```python
from build123d import *

# Parameters (mm, degrees)
ESQUISSE1_R             = 37
ESQUISSE1_R_2           = 1.5
ESQUISSE1_W             = 25
ESQUISSE1_H             = 3
BOSS_EXTRU_1_DEPTH      = 2
BOSS_EXTRU_2_DEPTH      = 15
ESQUISSE3_W             = 2
ESQUISSE3_H             = 28.4
BOSS_EXTRU_3_DEPTH      = 2.25
ESQUISSE5_W             = 2
ESQUISSE5_H             = 24.4
BOSS_EXTRU_4_DEPTH      = 2.25
ESQUISSE7_W             = 33.1
ESQUISSE7_H             = 28.4
BOSS_EXTRU_5_DEPTH      = 1
ESQUISSE8_W             = 15
ESQUISSE8_H             = 15
ENL_V_MAT_EXTRU_1_DEPTH = 3
ESQUISSE9_W             = 21
ESQUISSE9_H             = 2.5
ENL_V_MAT_EXTRU_2_DEPTH = 3
ESQUISSE10_R            = 1
ENL_V_MAT_EXTRU_3_DEPTH = 19
ESQUISSE11_W            = 33.1
ESQUISSE11_H            = 28.4
ENL_V_MAT_EXTRU_4_DEPTH = 15


with BuildPart() as part:
    # Esquisse1 → Boss.-Extru.1 (new body)
    with BuildSketch(Plane.XY):
        Circle(ESQUISSE1_R)
        with Locations((0, 30)):
            Circle(ESQUISSE1_R_2, mode=Mode.SUBTRACT)
        with Locations((-22.874807889, 14.34375)):
            Circle(ESQUISSE1_R_2, mode=Mode.SUBTRACT)
        with Locations((-25.416453209, -15.9375)):
            Circle(ESQUISSE1_R_2, mode=Mode.SUBTRACT)
        with Locations((0, -27)):
            Circle(ESQUISSE1_R_2, mode=Mode.SUBTRACT)
        with Locations((25.416453209, -15.9375)):
            Circle(ESQUISSE1_R_2, mode=Mode.SUBTRACT)
        with Locations((22.874807889, 14.34375)):
            Circle(ESQUISSE1_R_2, mode=Mode.SUBTRACT)
        with Locations((0, -15.5)):
            Rectangle(ESQUISSE1_W, ESQUISSE1_H, mode=Mode.SUBTRACT)
    extrude(amount=BOSS_EXTRU_1_DEPTH)

    # Esquisse2 → Boss.-Extru.2 (add)
    with BuildSketch(Plane(origin=(0, 0, 0), x_dir=(-1, 0, 0), z_dir=(0, 0, -1))):
        Polygon((-16.75, 14.9), (-12.75, 14.9), (-12.75, -9.5), (12.35, -9.5), (12.35, 14.9), (16.35, 14.9), (16.35, -13.5), (-16.75, -13.5), align=None)
    extrude(amount=BOSS_EXTRU_2_DEPTH)

    # Esquisse3 → Boss.-Extru.3 (add)
    with BuildSketch(Plane(origin=(-12.35, 0, 0), x_dir=(0, 0, -1), z_dir=(1, 0, 0))):
        with Locations((9.625, 0.7)):
            Rectangle(ESQUISSE3_W, ESQUISSE3_H)
        with Locations((6.625, 0.7)):
            Rectangle(ESQUISSE3_W, ESQUISSE3_H)
    extrude(amount=BOSS_EXTRU_3_DEPTH)

    # Esquisse5 → Boss.-Extru.4 (add)
    with BuildSketch(Plane.ZY.offset(-12.75)):
        with Locations((-9.625, 2.7)):
            Rectangle(ESQUISSE5_W, ESQUISSE5_H)
        with Locations((-6.625, 2.7)):
            Rectangle(ESQUISSE5_W, ESQUISSE5_H)
    extrude(amount=BOSS_EXTRU_4_DEPTH)

    # Esquisse7 → Boss.-Extru.5 (add)
    with BuildSketch(Plane(origin=(0, 0, -15), x_dir=(-1, 0, 0), z_dir=(0, 0, -1))):
        with Locations((-0.2, 0.7)):
            Rectangle(ESQUISSE7_W, ESQUISSE7_H)
    extrude(amount=-BOSS_EXTRU_5_DEPTH)

    # Esquisse8 → Enlèv. mat.-Extru.1 (cut)
    with BuildSketch(Plane(origin=(0, 0, -15), x_dir=(-1, 0, 0), z_dir=(0, 0, -1))):
        Rectangle(ESQUISSE8_W, ESQUISSE8_H)
    extrude(amount=-ENL_V_MAT_EXTRU_1_DEPTH, mode=Mode.SUBTRACT)

    # Esquisse9 → Enlèv. mat.-Extru.2 (cut)
    with BuildSketch(Plane.XZ.offset(13.5)):
        with Locations((0, -5.65)):
            Rectangle(ESQUISSE9_W, ESQUISSE9_H)
    extrude(amount=-ENL_V_MAT_EXTRU_2_DEPTH, mode=Mode.SUBTRACT)

    # Esquisse10 → Enlèv. mat.-Extru.3 (cut)
    with BuildSketch(Plane.XY.offset(2)):
        with Locations((-14.35, 8.9)):
            Circle(ESQUISSE10_R)
        with Locations((-14.35, -11.5)):
            Circle(ESQUISSE10_R)
        with Locations((14.75, -11.5)):
            Circle(ESQUISSE10_R)
        with Locations((14.75, 8.9)):
            Circle(ESQUISSE10_R)
    extrude(amount=-ENL_V_MAT_EXTRU_3_DEPTH, mode=Mode.SUBTRACT)

    # Esquisse11 → Enlèv. mat.-Extru.4 (cut)
    with BuildSketch(Plane(origin=(0, 0, -15), x_dir=(-1, 0, 0), z_dir=(0, 0, -1))):
        with Locations((-0.2, 0.7)):
            Rectangle(ESQUISSE11_W, ESQUISSE11_H)
    extrude(amount=-ENL_V_MAT_EXTRU_4_DEPTH, mode=Mode.SUBTRACT)


solid = part.part
```
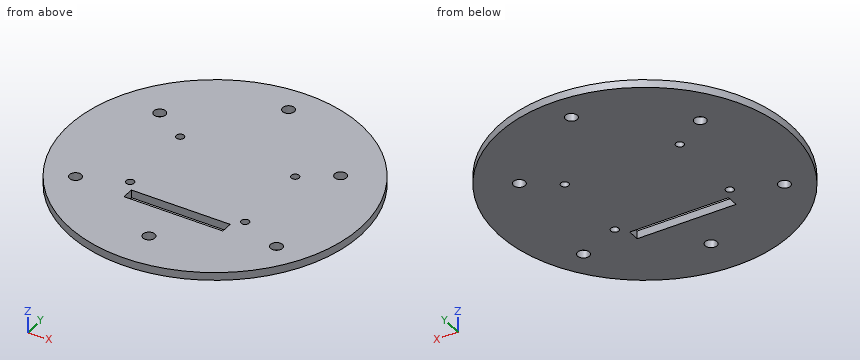
Can you work these out from the model? Positions are in its coordinate system, mm. Coordinates: 2 decimals unless noted, no trailing zeros. Write each loop counter-clockwise with the first axis right and the second up, starting at its lowest first coordinate (ties: lowest second). Pieces come first, ordered by that corner, then holes. Notation, with made-up numbers: M -22.5,29.5 L -6.5,29.5 A15 cw -6.5,49.5 Z; hole C 85.5,-34 d7. An arc over 180 degrees is marked long. Answer as CSV lines item,"result".
Item 1: Imagine slicing it at D-D on y = 30. List the corners of the cut face in (x, z) for me, plus the area to 3 significant figures.
Geometry results:
outline,"M -21.66,0 L -1.5,0 L -1.5,2 L -21.66,2 Z; M 1.5,0 L 21.66,0 L 21.66,2 L 1.5,2 Z"
area,"80.6 mm2"
Item 2: Imagine slicing it at B-B on y = 8.9. List the corners of the cut face in (x, z) for me, plus the area to 3 significant figures.
Geometry results:
outline,"M -35.91,0 L -15.35,0 L -15.35,2 L -35.91,2 Z; M -13.35,0 L 13.75,0 L 13.75,2 L -13.35,2 Z; M 15.75,0 L 35.91,0 L 35.91,2 L 15.75,2 Z"
area,"136 mm2"
Item 3: Imagine slicing it at C-C on x = -14.35. List the corners of the cut face in (y, z) for me.
Geometry results:
outline,"M -34.1,0 L -12.5,0 L -12.5,2 L -34.1,2 Z; M -10.5,0 L 7.9,0 L 7.9,2 L -10.5,2 Z; M 9.9,0 L 34.1,0 L 34.1,2 L 9.9,2 Z"
Item 4: I'm going to push flat-ended pins straight in: P1, Ø0.6, axis at x = 3, z = 1, coming from the -Y side; P2, Ø2.5, axis at x = 0, y = 30, coming from the +Z side; P3, Ø1, axis at y = -9.5, z = 2, coming from the +X side; P4, Ø0.6, axis at y = -16, z = 1, coming from the +X side. Where does each tip first touch, or does it pass through?
Geometry results:
P1,"stops at y = -36.9"
P2,"passes through"
P3,"stops at x = 35.89"
P4,"stops at x = 33.5"
Item 5: Please list where these lines run through material, in increasing order: line 1 along Y through (x, z) = (0, 1.05); line 2 along X through (y, z) = (13, 1.8); line 3 along Y through (x, z) = (-0.5, 1.3).
Geometry results:
line 1,"y = -37 to -28.5, -25.5 to -17, -14 to 28.5, 31.5 to 37"
line 2,"x = -34.64 to -23.54, -22.21 to 22.21, 23.54 to 34.64"
line 3,"y = -37 to -28.41, -25.59 to -17, -14 to 28.59, 31.41 to 37"
Item 6: Imagine slicing it at A-A on x = 0. List the corners of the cut face in (y, z) for me.
Geometry results:
outline,"M -37,0 L -28.5,0 L -28.5,2 L -37,2 Z; M -25.5,0 L -17,0 L -17,2 L -25.5,2 Z; M -14,0 L 28.5,0 L 28.5,2 L -14,2 Z; M 31.5,0 L 37,0 L 37,2 L 31.5,2 Z"
